Source: CAD feature listing. Evaluate the final solid. Frame: model axes, mm. Face numbers are marked on the shaded views. A direction names the side the tool comes from. Give positions to 0.01 mm unless a question says otherwise; leave off trailing zeros. Order: outer loops, then holes, each group sorted by start corner. A loop starts at its lowest first (then second) coordinate and runs counter-clockwise, first axis right, second up. Notation, with made-up numbers: (87, 57.5) - (135, 57.5) arc R8 ccw to (135, 68.5) - close; hole circle Ø2 at (84, 20.5). An arc over 180 degrees is marked (long way). One line per item, written item: value. Start each with the question number.
from build123d import *

# Parameters (mm, degrees)
SKETCH1_R           = 35
SKETCH1_W           = 3.2
SKETCH1_H           = 5.2
BOSS_EXTRUDE1_DEPTH = 2
SKETCH2_W           = 7.2
SKETCH2_H           = 9.2
SKETCH2_W_2         = 3.2
SKETCH2_H_2         = 5.2
BOSS_EXTRUDE2_DEPTH = 3
SKETCH3_W           = 4
SKETCH3_H           = 50
BOSS_EXTRUDE3_DEPTH = 50
SKETCH4_R           = 3.1
SKETCH4_R_2         = 2.1
CUT_EXTRUDE1_DEPTH  = 50
FILLET1_R           = 20
SKETCH6_W           = 10
SKETCH6_H           = 4
BOSS_EXTRUDE4_DEPTH = 15
CUT_EXTRUDE2_DEPTH  = 15
SKETCH8_R           = 7.889109842
CUT_EXTRUDE3_DEPTH  = 2
SKETCH9_R           = 10
SKETCH9_W           = 7.2
SKETCH9_H           = 9.2
BOSS_EXTRUDE5_DEPTH = 3


with BuildPart() as part:
    # Sketch1 → Boss-Extrude1 (new body)
    with BuildSketch(Plane(origin=(0, 0, 0), x_dir=(1, 0, 0), z_dir=(0, 1, 0))):
        with Locations(Location((0, 0, 0), (0, 0, 270))):
            Circle(SKETCH1_R)
        Rectangle(SKETCH1_W, SKETCH1_H, mode=Mode.SUBTRACT)
    extrude(amount=BOSS_EXTRUDE1_DEPTH)

    # Sketch2 → Boss-Extrude2 (add)
    with BuildSketch(Plane.XZ):
        Rectangle(SKETCH2_W, SKETCH2_H)
        Rectangle(SKETCH2_W_2, SKETCH2_H_2, mode=Mode.SUBTRACT)
    extrude(amount=BOSS_EXTRUDE2_DEPTH)

    # Sketch3 → Boss-Extrude3 (add)
    with BuildSketch(Plane(origin=(0, 2, 0), x_dir=(1, 0, 0), z_dir=(0, 1, 0))):
        with Locations((-9.6, 0)):
            Rectangle(SKETCH3_W, SKETCH3_H)
    extrude(amount=BOSS_EXTRUDE3_DEPTH)

    # Sketch4 → Cut-Extrude1 (cut)
    with BuildSketch(Plane(origin=(-7.6, 0, 0), x_dir=(0, 0, -1), z_dir=(1, 0, 0))):
        with Locations((0, 33.691273446)):
            Circle(SKETCH4_R)
        with Locations((-18, 25.191273446)):
            Circle(SKETCH4_R_2)
        with Locations((18, 25.191273446)):
            Circle(SKETCH4_R_2)
    extrude(amount=-CUT_EXTRUDE1_DEPTH, mode=Mode.SUBTRACT)

    # Fillet1
    fillet1_edges = [part.edges().sort_by_distance(p)[0] for p in [
        (-9.6, 52, 25),
        (-9.6, 52, -25),
    ]]
    fillet(fillet1_edges, radius=FILLET1_R)

    # Sketch6 → Boss-Extrude4 (add)
    with BuildSketch(Plane(origin=(0, 2, 0), x_dir=(1, 0, 0), z_dir=(0, 1, 0))):
        with Locations((-16.6, -23)):
            Rectangle(SKETCH6_W, SKETCH6_H)
    extrude(amount=BOSS_EXTRUDE4_DEPTH)

    # Sketch7 → Cut-Extrude2 (cut)
    with BuildSketch(Plane.XY.offset(25)):
        Polygon((-11.6, 2), (-11.6, 17), (-15.110464725, 17), (-15.110464725, 14.98052876), (-19.421422774, 10.669570711), (-19.421422774, 2), align=None)
    extrude(amount=-CUT_EXTRUDE2_DEPTH, mode=Mode.SUBTRACT)

    # Sketch8 → Cut-Extrude3 (cut)
    with BuildSketch(Plane(origin=(-7.6, 0, 0), x_dir=(0, 0, -1), z_dir=(1, 0, 0))):
        with Locations((0, 33.691273446)):
            Circle(SKETCH8_R)
    extrude(amount=-CUT_EXTRUDE3_DEPTH, mode=Mode.SUBTRACT)

    # Sketch9 → Boss-Extrude5 (add)
    with BuildSketch(Plane.XZ.offset(3)):
        with Locations(Location((0, 0, 0), (0, 0, 270))):
            Circle(SKETCH9_R)
        Rectangle(SKETCH9_W, SKETCH9_H, mode=Mode.SUBTRACT)
    extrude(amount=-BOSS_EXTRUDE5_DEPTH)


solid = part.part
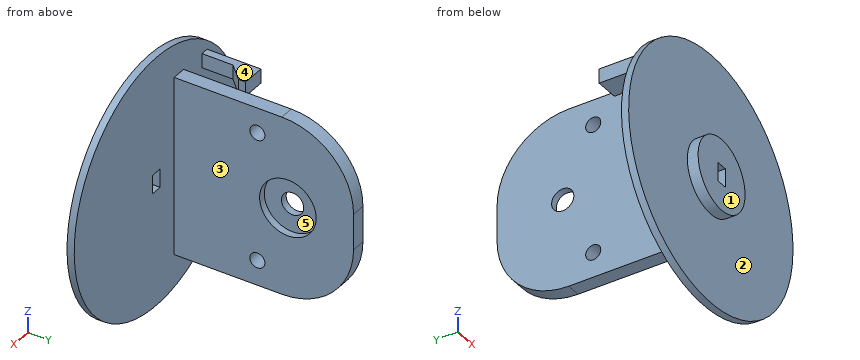
1. Section D-D on z = 27. Return the cut outline in (x, y).
2. Contact query for flat-ended pins moving along their axis: pin 1 Ø10 at (x, z) = (7, 14) entering from +Y; pin 2 Ø1.5 at (y, z) = (27.5, 21) entering from +X; pin 3 Ø10 at (y, z) = (42.5, -21) entering from -X. Output: stop coordinate, or through.
3. Section C-C on z = 18. Return the cut outline in (x, y).
4. Section A-A on x = 0. Return the cut outline in (y, z), then the cut area to 3 significant figures.
5. Set-up query: the marked faces 1 and 2. Return all of +Z, -Z, +X, -X, +Y, -Y with unobstructed straight access to the full face (end or side cutting, diameter ignored); none if empty.
6. Ray query, L1, parallel to X at y = 2.5, z = 21.5; L2, parallel to Y at x = -8.25, z = 0; L3, parallel to X at y = 28.5, z = 3.5. Return the intervals inside material, ascending.
7. Draft query along Z for the marked faces 3, 4 and 5. Return one class per face: pulls with the +Z half, pulls with the -Z half, needs draft (parallel to the pull), parting line crosses it, or undercut.
8. Section B-B on z = 0. Return the cut outline in (x, y).
Data:
1. outline: (-22.27, 0) - (22.27, 0) - (22.27, 2) - (-22.27, 2) - close
2. pin 1: stops at y = 2
2. pin 2: stops at x = -7.6
2. pin 3: stops at x = -11.6
3. outline: (-30.02, 0) - (30.02, 0) - (30.02, 2) - (-7.6, 2) - (-7.6, 23.09) - (-11.6, 23.09) - (-11.6, 2) - (-30.02, 2) - close; (-11.6, 27.29) - (-7.6, 27.29) - (-7.6, 47.2) - (-11.6, 47.2) - close
4. outline: (-3, -10) - (0, -10) - (0, -35) - (2, -35) - (2, -2.6) - (-3, -2.6) - close; (-3, 2.6) - (2, 2.6) - (2, 35) - (0, 35) - (0, 10) - (-3, 10) - close
4. area: 174 mm2
5. face 1: +Z, -Z, +X, -X, -Y
5. face 2: -Y
6. L1: x = -21.6 to -19.42, -11.6 to -7.6
6. L2: y = -3 to 25.8, 41.58 to 52
6. L3: x = -11.6 to -9.6
7. face 3: needs draft
7. face 4: pulls with the +Z half
7. face 5: undercut
8. outline: (-35, 0) - (-10, 0) - (-10, -3) - (-1.6, -3) - (-1.6, 2) - (-7.6, 2) - (-7.6, 25.8) - (-9.6, 25.8) - (-9.6, 30.59) - (-11.6, 30.59) - (-11.6, 2) - (-35, 2) - close; (-11.6, 36.79) - (-9.6, 36.79) - (-9.6, 41.58) - (-7.6, 41.58) - (-7.6, 52) - (-11.6, 52) - close; (1.6, -3) - (10, -3) - (10, 0) - (35, 0) - (35, 2) - (1.6, 2) - close
